Print and shaded views of the part. All mm, measured from the part's lowest x, y and z. Give positions to 0.01 mm unless a question says otherwise; leave off trailing zeros. Loops run counter-clockwise (first coordinate to the right, second up) from the corner with the lowest first, then second, coordinate; pieces in that order, holes last. Notation, with made-up numbers: (16.5, 38.5) -> (60.5, 38.5) arc R19 cw to (60.5, 47.5) -> close; hole circle Ø10 at (-22, 73). An arc over 180 degrees is marked (long way). Write each question's results on one line, items separated by ' | '. Start each with the question number.
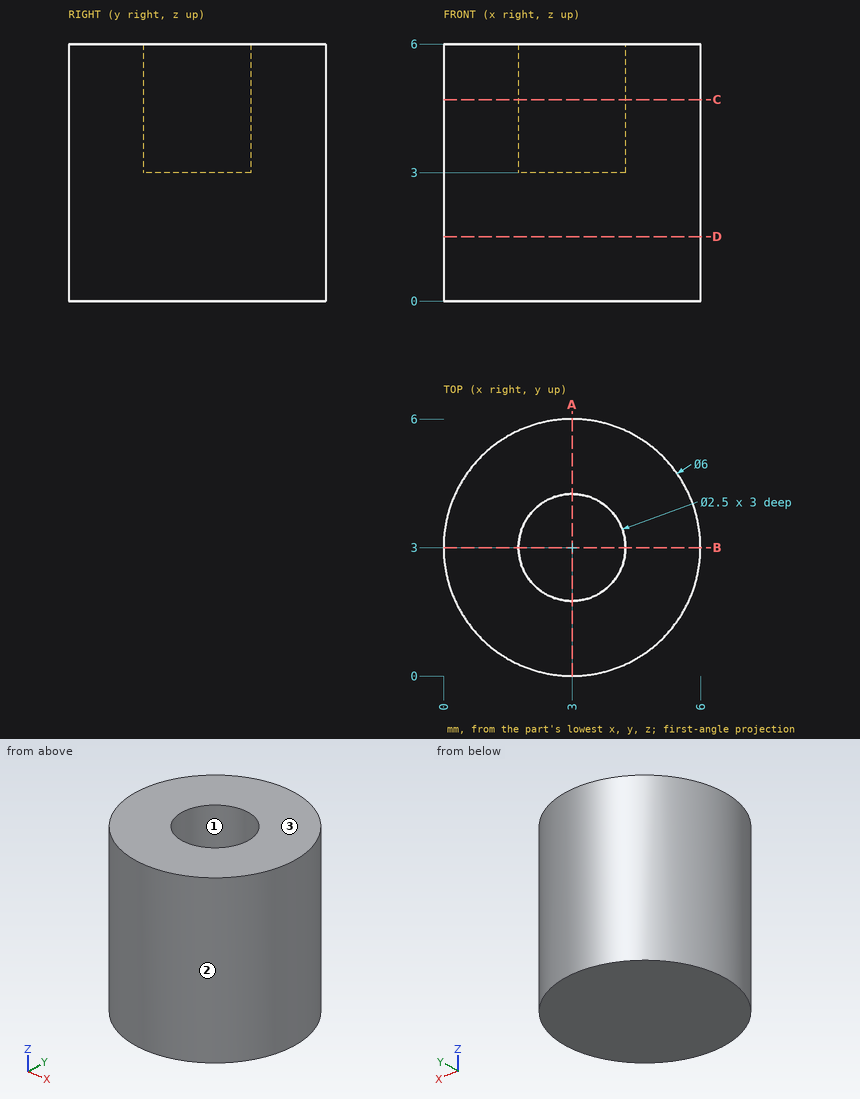
Q1. Saw through at A-A, the plane x = 3. List the corners of the cut face in (y, z).
Q2. Wall check: L1, parallel to Y at x = 3, z = 4.95; L2, parallel to Z at x = 3.85, y = 3; L3, parallel to X at y = 5.15, z = 1.85. Give the ranges that are in metal, low to high.
Q3. Mould opens along Y. For the marked faces 1, 2 and 3 say: pulls with the +Y half, pulls with the -Y half, needs draft (parallel to the pull), parting line crosses it, or undercut.
Q4. Saw through at C-C, the plane z = 4.7. List the corners of the cut face in (x, y).
Q5. Drop flat-ended pins along their axis: pin 1 (1.5 mm diameter, centred on y = 2, z = 1.5, fed in from -X); pin 2 (2 mm diameter, centred on x = 3, y = 3, fed in from +Z). Give the stop position or say it passes through.
Q6. Saw through at D-D, the plane z = 1.5. List the corners of the cut face in (x, y).
Answer block:
1) outline: (0, 0) -> (6, 0) -> (6, 6) -> (4.25, 6) -> (4.25, 3) -> (1.75, 3) -> (1.75, 6) -> (0, 6) -> close
2) L1: y = 0 to 1.75, 4.25 to 6 | L2: z = 0 to 3 | L3: x = 0.91 to 5.09
3) face 1: undercut | face 2: parting line crosses it | face 3: needs draft
4) outline: circle Ø6 at (3, 3); hole circle Ø2.5 at (3, 3)
5) pin 1: stops at x = 0.01 | pin 2: stops at z = 3
6) outline: circle Ø6 at (3, 3)
